```python
from build123d import *

# Parameters (mm, degrees)
ESBO_O4_W                  = 92
ESBO_O4_H                  = 99.397000359
RESSALTO_EXTRUS_O2_DEPTH   = 0.8
CORTE_EXTRUS_O1_START      = -1
CORTE_EXTRUS_O1_DEPTH      = 1
CORTE_EXTRUS_O2_DEPTH      = 136.212783118
FILETE8_R                  = 1
CORTE_EXTRUS_O4_DEPTH      = 136.212783118
CORTE_EXTRUS_O4_DEPTH_BACK = 136.212783118
FILETE10_R                 = 2
FILETE11_R                 = 3


with BuildPart() as part:
    # Varredura1: sweep along a path in Esboço1
    with BuildLine(Plane.XY) as varredura1_path:
        Line((0, 0), (0, 69.096427937))
        ThreePointArc((0, 69.096427937), (-4.342158003, 81.53957802), (-15.483198399, 88.579715732))
        ThreePointArc((-15.483198399, 88.579715732), (-46, 92.070770961), (-76.516801601, 88.579715732))
        ThreePointArc((-76.516801601, 88.579715732), (-87.657841997, 81.53957802), (-92, 69.096427937))
        Line((-92, 69.096427937), (-92, 0))
    # Esboço2 → Varredura1 (sweep)
    with BuildSketch(Plane(origin=(0, 0, 0), x_dir=(1, 0, 0), z_dir=(0, 1, 0))):
        with BuildLine():
            Line((-0.8, -28.273328944), (-0.09293029, -32.044242141))
            Line((-0.09293029, -32.044242141), (-0.830714704, -28.401410992))
            Line((-0.830714704, -28.401410992), (-1.53336923, -28.543719964))
            Line((-1.53336923, -28.543719964), (-0.8, -32.044242141))
            ThreePointArc((-0.8, -32.044242141), (-0.092135156, -32.613021625), (0.75, -32.273328944))
            Line((0.75, -32.273328944), (0, -28.273328944))
            Line((0, -28.273328944), (0, 0))
            Line((0, 0), (-0.8, 0))
            Line((-0.8, 0), (-0.8, -28.273328944))
        make_face()
    sweep(path=varredura1_path.line)

    # Esboço4 → Ressalto-extrusão2 (add)
    with BuildSketch(Plane(origin=(0, 0, 0), x_dir=(-1, 0, 0), z_dir=(0, 0, -1))):
        with Locations((46, 49.69850018)):
            Rectangle(ESBO_O4_W, ESBO_O4_H)
    extrude(amount=-RESSALTO_EXTRUS_O2_DEPTH)

    # Esboço6 → Corte-extrusão1 (cut)
    with BuildSketch(Plane.XY.offset(0.8).offset(CORTE_EXTRUS_O1_START)):
        with BuildLine():
            Line((-92, 69.096427937), (-92, 105.833978266))
            Line((-92, 105.833978266), (0, 105.833978266))
            Line((0, 105.833978266), (0, 69.096427937))
            ThreePointArc((0, 69.096427937), (-4.342158003, 81.53957802), (-15.483198399, 88.579715732))
            ThreePointArc((-15.483198399, 88.579715732), (-46, 92.070770961), (-76.516801601, 88.579715732))
            ThreePointArc((-76.516801601, 88.579715732), (-87.657841997, 81.53957802), (-92, 69.096427937))
        make_face()
    extrude(amount=CORTE_EXTRUS_O1_DEPTH, mode=Mode.SUBTRACT)

    # Esboço7 → Corte-extrusão2 (cut, through all)
    with BuildSketch(Plane(origin=(0, 0, 0), x_dir=(-1, 0, 0), z_dir=(0, 0, -1))):
        with BuildLine():
            Line((55.9, 53.55), (55.9, 33.75))
            ThreePointArc((55.9, 33.75), (46, 29.734257245), (36.1, 33.75))
            Line((36.1, 33.75), (36.1, 53.55))
            ThreePointArc((36.1, 53.55), (46, 57.565742755), (55.9, 53.55))
        make_face()
    extrude(amount=-CORTE_EXTRUS_O2_DEPTH, mode=Mode.SUBTRACT)

    # Filete8
    # the kernel refuses this fillet: 1 mm, written as the material it takes off along each edge
    with BuildSketch(Plane(origin=(-46, -43.054940969, 28.543719964), x_dir=(0.22584008006616485, 0.9741643897390769, 0), z_dir=(0.9741643897390769, -0.22584008006616485, 0))) as filete8_piece_1:
        with BuildLine():
            CenterArc((134.768740044, 0.738354268), FILETE8_R, 168.167507323, 73.554966167)
            Line((133.789988783, 0.943405407), (133.770413758, 0.947506429))
            Line((133.770413758, 0.947506429), (133.572767675, 0.004101023))
            Line((133.572767675, 0.004101023), (133.588372694, -0.019602016))
            ThreePointArc((133.588372694, -0.019602016), (133.939699957, -0.090756503), (134.28552237, -0.159922237))
            Line((134.28552237, -0.159922237), (134.294997227, -0.142308972))
        make_face()
    revolve(axis=Axis((-46, -43.054940969, 28.543719964), (0, 0, 1)), revolution_arc=26.104565599, mode=Mode.SUBTRACT)
    with BuildSketch(Plane(origin=(-72, 69.096427937, 28.543719964), x_dir=(-0.2258400800661638, 0.9741643897390773, 0), z_dir=(0.9741643897390773, 0.2258400800661638, 0))) as filete8_piece_2:
        with BuildLine():
            CenterArc((19.643028114, 0.738354268), FILETE8_R, 168.167507323, 73.554966167)
            Line((19.169285296, -0.142308972), (19.15981044, -0.159922237))
            ThreePointArc((19.15981044, -0.159922237), (18.813988027, -0.090756503), (18.462660764, -0.019602016))
            Line((18.462660764, -0.019602016), (18.447055745, 0.004101023))
            Line((18.447055745, 0.004101023), (18.644701828, 0.947506429))
            Line((18.644701828, 0.947506429), (18.664276853, 0.943405407))
        make_face()
    revolve(axis=Axis((-72, 69.096427937, 28.543719964), (0, 0, 1)), revolution_arc=76.9477172, mode=Mode.SUBTRACT)
    with BuildSketch(Plane(origin=(-90.46663077, 69.096427937, 28.543719964), x_dir=(-0.20505113872706254, 0, 0.9787512607944548), z_dir=(0, -1, 0))) as filete8_piece_3:
        with BuildLine():
            CenterArc((0.963886786, 1), FILETE8_R, 196.445033833, 73.554966167)
            Line((0.004795025, 0.716904621), (-0.014386811, 0.711242713))
            ThreePointArc((-0.014386811, 0.711242713), (-0.01760204, 0.358586078), (-0.019999553, 0.000133767))
            Line((-0.019999553, 0.000133767), (0, -0.02))
            Line((0, -0.02), (0.963886786, -0.02))
            Line((0.963886786, -0.02), (0.963886786, 0))
        make_face()
    extrude(amount=71.506144901, mode=Mode.SUBTRACT)
    with BuildSketch(Plane(origin=(-20, 69.096427937, 28.543719964), x_dir=(1, 0, 0), z_dir=(0, -1, 0))) as filete8_piece_4:
        with BuildLine():
            CenterArc((19.643028114, 0.738354268), FILETE8_R, 168.167507323, 73.554966167)
            Line((18.664276853, 0.943405407), (18.644701828, 0.947506429))
            Line((18.644701828, 0.947506429), (18.447055745, 0.004101023))
            Line((18.447055745, 0.004101023), (18.462660764, -0.019602016))
            ThreePointArc((18.462660764, -0.019602016), (18.813988027, -0.090756503), (19.15981044, -0.159922237))
            Line((19.15981044, -0.159922237), (19.169285296, -0.142308972))
        make_face()
    revolve(axis=Axis((-20, 69.096427937, 28.543719964), (0, 0, 1)), revolution_arc=76.9477172, mode=Mode.SUBTRACT)
    with BuildSketch(Plane(origin=(-1.53336923, -2.409716964, 28.543719964), x_dir=(0.9801008248789868, 0, -0.19850031000361154), z_dir=(0, 1, 0))) as filete8_piece_5:
        with BuildLine():
            CenterArc((1.006424456, -0.957176864), FILETE8_R, 106.828251577, 73.554966167)
            Line((0.006446823, -0.963865226), (-0.013552729, -0.963998993))
            Line((-0.013552729, -0.963998993), (-0.019999553, -0.000133767))
            Line((-0.019999553, -0.000133767), (0, 0.02))
            ThreePointArc((0, 0.02), (0.358460328, 0.02), (0.71113058, 0.019143537))
            Line((0.71113058, 0.019143537), (0.716920656, 0))
        make_face()
    extrude(amount=71.506144901, mode=Mode.SUBTRACT)

    # Esboço8 → Corte-extrusão4 (cut, two sides: drawn at the far end of the back side and taken through both)
    with BuildSketch(Plane(origin=(0, 0, 0), x_dir=(0, 0, -1), z_dir=(1, 0, 0)).offset(-CORTE_EXTRUS_O4_DEPTH_BACK)):
        with BuildLine():
            Line((-14.136664472, 0), (-28.273328944, 0))
            ThreePointArc((-28.273328944, 0), (-31.102110178, 1.288762683), (-32.622670844, 4))
            Line((-32.622670844, 4), (-38.469837325, 4))
            Line((-38.469837325, 4), (-38.469837325, -4.573477319))
            Line((-38.469837325, -4.573477319), (-14.136664472, -4.573477319))
            Line((-14.136664472, -4.573477319), (-14.136664472, 0))
        make_face()
    extrude(amount=CORTE_EXTRUS_O4_DEPTH + CORTE_EXTRUS_O4_DEPTH_BACK, mode=Mode.SUBTRACT)

    # Filete10
    filete10_edges = [part.edges().sort_by_distance(p)[0] for p in [
        (-0.8, 34.548213968, 0.8),
        (-91.2, 34.548213968, 0.8),
        (-87.031528317, 81.041852016, 0.8),
        (-46, 91.270770961, 0.8),
        (-4.968471683, 81.041852016, 0.8),
    ]]
    fillet(filete10_edges, radius=FILETE10_R)

    # Filete11
    filete11_edges = [part.edges().sort_by_distance(p)[0] for p in [
        (0, 34.548213968, 0),
        (-92, 34.548213968, 0),
        (-87.657841997, 81.53957802, 0),
        (-4.342158003, 81.53957802, 0),
        (-46, 92.070770961, 0),
    ]]
    fillet(filete11_edges, radius=FILETE11_R)


solid = part.part
```
Design review of the part built by this model. Coordinates are the model's own, in mm. A direction names the side the tool comes from. Round coordinates to 2 decimals unless told otherwise and drop trailing zeros. Write each loop counter-clockwise with the first axis right and the second up, starting at its lowest first coordinate (ties: lowest second). Pieces come first, ordered by that corner, then holes. Notation, with made-up numbers: (9, -23.5) -> (45, -23.5) arc R10 cw to (45, -14.5) -> close; hole circle Ø4 at (75.25, 80.25). An arc over 180 degrees is marked (long way). Answer in a Markdown table with one row per item.
Q1. Take a section at C-C, the plane y = 66. State the section outline as (x, z) points, then the cut area to 3 significant figures.
The answers:
| item | result |
|---|---|
| outline | (-92.75, 32.27) -> (-92, 28.27) -> (-92, 3) arc R3 ccw to (-89, 0) -> (-3, 0) arc R3 ccw to (0, 3) -> (0, 28.27) -> (0.75, 32.27) arc R0.9 ccw to (-0.8, 32.04) -> (-1.34, 29.49) arc R1 ccw to (-0.83, 28.4) -> (-0.09, 32.04) -> (-0.8, 28.27) -> (-0.8, 2.8) arc R2 cw to (-2.8, 0.8) -> (-89.2, 0.8) arc R2 cw to (-91.2, 2.8) -> (-91.2, 28.27) -> (-91.91, 32.04) -> (-91.17, 28.4) arc R1 ccw to (-90.66, 29.49) -> (-91.2, 32.04) arc R0.9 ccw to start |
| area | 128 mm² |
Q2. Take a section at A-A, the plane y = 49.5. State the section outline as (x, z) points, then the cut area to 3 significant figures.
The answers:
| item | result |
|---|---|
| outline | (-92.75, 32.27) -> (-92, 28.27) -> (-92, 3) arc R3 ccw to (-89, 0) -> (-55.9, 0) -> (-55.9, 0.8) -> (-89.2, 0.8) arc R2 cw to (-91.2, 2.8) -> (-91.2, 28.27) -> (-91.91, 32.04) -> (-91.17, 28.4) arc R1 ccw to (-90.66, 29.49) -> (-91.2, 32.04) arc R0.9 ccw to start; (-36.1, 0) -> (-3, 0) arc R3 ccw to (0, 3) -> (0, 28.27) -> (0.75, 32.27) arc R0.9 ccw to (-0.8, 32.04) -> (-1.34, 29.49) arc R1 ccw to (-0.83, 28.4) -> (-0.09, 32.04) -> (-0.8, 28.27) -> (-0.8, 2.8) arc R2 cw to (-2.8, 0.8) -> (-36.1, 0.8) -> close |
| area | 112 mm² |
Q3. For faces 1 (the face through (-90.93, 34.21, 30.75)), 2 (the face through (-91.2, 34, 15)), 3 (the face through (-92.38, 34.06, 30.3)), list the 3-axis set-ups (+Z, -Z, +X, -X, +Y, -Y) from which the entire face can be reached by the end or side of a thin tool; tool diameter is ignored.
The answers:
| item | result |
|---|---|
| face 1 | +Z, -Y |
| face 2 | -Y |
| face 3 | -Z, -X, +Y, -Y |
Q4. Draft analysis for pull direction Y (two halves, no side actions). For faces 4 (the face through (0, 35, 16)), 5 (the face through (-45.847, 57.565, 0.394)), 6 (the face through (-4.226, 81.392, 15.46)), 7 (the face through (-46.153, 29.735, 0.394)), state which applies: +Y half, -Y half, draft (parallel to the pull), parting line (faces both ways), or undercut.
The answers:
| item | result |
|---|---|
| face 4 | draft |
| face 5 | undercut |
| face 6 | +Y half |
| face 7 | undercut |
Q5. Take a section at B-B, the plane z = 24.5. State the section outline as (x, y) points, then the cut area to 3 significant figures.
The answers:
| item | result |
|---|---|
| outline | (-92, 0) -> (-91.2, 0) -> (-91.2, 69.1) arc R19.2 cw to (-76.34, 87.8) arc R134.33 cw to (-15.66, 87.8) arc R19.2 cw to (-0.8, 69.1) -> (-0.8, 0) -> (0, 0) -> (0, 69.1) arc R20 ccw to (-15.48, 88.58) arc R135.13 ccw to (-76.52, 88.58) arc R20 ccw to (-92, 69.1) -> close |
| area | 202 mm² |
Q6. To check wall thickness, follow L1, parallel to X at y = 40.5, z = 3; L2, parallel to Z at x = -70, y = 6.5; L3, parallel to Y at x = -76.5, z = 9.5. State the ranges of each line that lie inside material, in increasing order. Write a range as [from, to].
The answers:
| item | result |
|---|---|
| L1 | [-92, -91.2], [-0.8, 0] |
| L2 | [0, 0.8] |
| L3 | [87.76, 88.58] |
Q7. Clearance check with flat-ended pins moving along their axes: pin 1 Ø1.5 at (x, y) = (-24, 20) entering from +Z; pin 2 Ø5 at (y, z) = (52.5, 4.5) entering from +X; pin 3 Ø0.6 at (y, z) = (43, 0.5) entering from -X; pin 4 Ø5 at (x, y) = (-36.5, 52.5) entering from -Z. State where each tip first meets the part, or that it passes through.
The answers:
| item | result |
|---|---|
| pin 1 | z = 0.8 |
| pin 2 | x = 0 |
| pin 3 | x = -91.04 |
| pin 4 | z = 0 |
